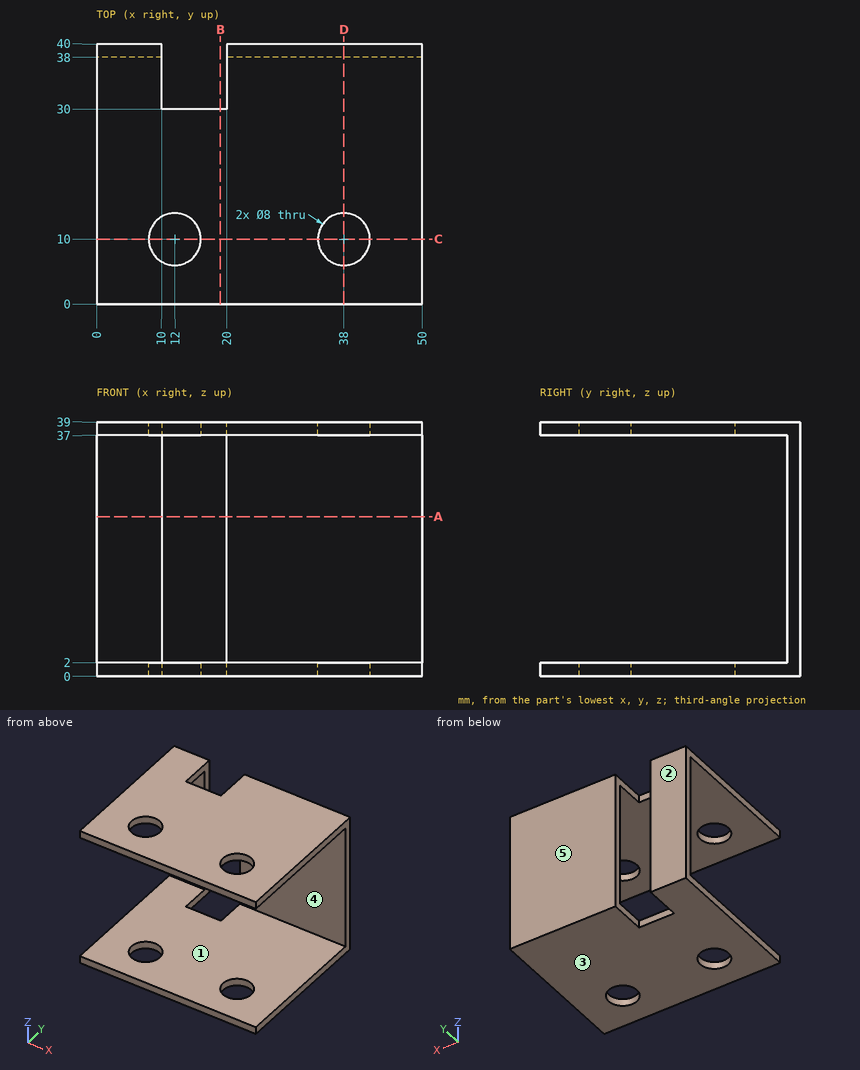
Print and shaded views of the part. All mm, measured from the part's lowest x, y and z. A direction names the side the tool comes from. Give positions to 0.01 mm unless a question says otherwise; leave off trailing zeros. Loops run counter-clockwise (first coordinate to the right, second up) from the corner with the lowest first, then second, coordinate; pieces in that order, holes last. Notation, with made-up numbers: (27.25, 66.5) - (73.25, 66.5) arc R26 ccw to (73.25, 81.5) - close; hole circle Ø3 at (39.25, 58.25). An arc over 180 degrees is marked (long way). One line per item, written item: value. Start each with the question number.
1. Slice it at D-D (x = 38). List the corners of the cut face in (y, z).
2. Pin check, flat tips, straight feed: pin 1 (12 mm diameter, centred on x = 8, z = 13.5, fed in from -Y); pin 2 (1.6 mm diameter, centred on x = 16, z = 1, fed in from +Y). Stop position of each tip, or through.
3. Probe L1, parallel to Y at x = 38, z = 37.6; L2, parallel to Z at x = 35, y = 17; L3, parallel to Y at x = 12, z = 38.35. List the from-to ranges inside material, lowest first. Write a range as from..to.
4. Pull direction Z, two halves, no side cores. Call the marked faces 3, 4 and 5: pulls with the +Z half, pulls with the -Z half, needs draft (parallel to the pull), parting line crosses it, or undercut.
5. Which spindle directions (+Z, -Z, +X, -X, +Y, -Y) get a long thin tool onto all of the face, cutting with end or side? Do the marked faces 1 and 2. Say none if no direction does.
6. Slice it at C-C (y = 10). List the corners of the cut face in (x, z), plus the area to 3 significant figures.
7. Slice it at B-B (x = 19). List the corners of the cut face in (y, z), plus the area to 3 significant figures.
8. Slice it at A-A (z = 24.5). List the corners of the cut face in (x, y), plus the area to 3 significant figures.
Solution:
1. outline: (0, 0) - (6, 0) - (6, 2) - (0, 2) - close; (0, 37) - (6, 37) - (6, 39) - (0, 39) - close; (14, 0) - (40, 0) - (40, 39) - (14, 39) - (14, 37) - (38, 37) - (38, 2) - (14, 2) - close
2. pin 1: stops at y = 38
2. pin 2: stops at y = 30
3. L1: y = 0..6, 14..40
3. L2: z = 0..2, 37..39
3. L3: y = 0..6, 14..30
4. face 3: pulls with the -Z half
4. face 4: undercut
4. face 5: needs draft
5. face 1: +X, -X, -Y
5. face 2: +Z, -Z, +X, -X, +Y
6. outline: (0, 0) - (8, 0) - (8, 2) - (0, 2) - close; (0, 37) - (8, 37) - (8, 39) - (0, 39) - close; (16, 0) - (34, 0) - (34, 2) - (16, 2) - close; (16, 37) - (34, 37) - (34, 39) - (16, 39) - close; (42, 0) - (50, 0) - (50, 2) - (42, 2) - close; (42, 37) - (50, 37) - (50, 39) - (42, 39) - close
6. area: 136 mm^2
7. outline: (0, 0) - (30, 0) - (30, 2) - (0, 2) - close; (0, 37) - (30, 37) - (30, 39) - (0, 39) - close
7. area: 120 mm^2
8. outline: (0, 38) - (10, 38) - (10, 40) - (0, 40) - close; (20, 38) - (50, 38) - (50, 40) - (20, 40) - close
8. area: 80.0 mm^2
